Geometry: final body of the model. Coordinates: model frame, mm. Give positions to 0.01 mm unless a question says otherwise; leave off trailing zeros. Write each loop counter-clockwise with the first axis right and the second up, starting at its lowest first coordinate (ties: lowest second). Pieces come first, ordered by that corner, then holes. Notation, with made-up numbers: M 62.25,70 L 104.25,70 A30 ccw 104.25,104 Z; hole C 18,-12 d5. An arc over 180 degrees is marked long. One line per question, with ' | ' between items.
from build123d import *

# Parameters (mm, degrees)
F0_W     = 100
F0_H     = 120
F0_R     = 2
F1_DEPTH = 2
F3_DEPTH = 25
F4_R     = 1.5
F5_DEPTH = 2.001


with BuildPart() as f1:
    # F0 (on Front) → F1 (new body)
    with BuildSketch(Plane.XZ):
        Rectangle(F0_W, F0_H)
        with Locations((-40, -50)):
            Circle(F0_R, mode=Mode.SUBTRACT)
        with Locations((40, -50)):
            Circle(F0_R, mode=Mode.SUBTRACT)
        with Locations((-40, 50)):
            Circle(F0_R, mode=Mode.SUBTRACT)
        with Locations((40, 50)):
            Circle(F0_R, mode=Mode.SUBTRACT)
    extrude(amount=F1_DEPTH)

    # F2 (on face) → F3 (cut)
    with BuildSketch(Plane.XZ.offset(2)):
        with BuildLine():
            Line((-1.25, 21.980018), (-9.75, 17.072541))
            ThreePointArc((-9.75, 17.072541), (-10.665064, 16.157477), (-11, 14.907477))
            Line((-11, 14.907477), (-11, 5.092523))
            ThreePointArc((-11, 5.092523), (-10.665064, 3.842523), (-9.75, 2.927459))
            Line((-9.75, 2.927459), (-1.25, -1.980018))
            ThreePointArc((-1.25, -1.980018), (0, -2.314955), (1.25, -1.980018))
            Line((1.25, -1.980018), (9.75, 2.927459))
            ThreePointArc((9.75, 2.927459), (10.665064, 3.842523), (11, 5.092523))
            Line((11, 5.092523), (11, 10.354255))
            Line((11, 10.354255), (0, 10.354255))
            Line((0, 10.354255), (0, 22.314955))
            ThreePointArc((0, 22.314955), (-0.647048, 22.229769), (-1.25, 21.980018))
        make_face()
        with BuildLine():
            ThreePointArc((1.25, 21.980018), (0.647048, 22.229769), (0, 22.314955))
            Line((0, 22.314955), (0, 10.354255))
            Line((0, 10.354255), (11, 10.354255))
            Line((11, 10.354255), (11, 14.907477))
            ThreePointArc((11, 14.907477), (10.665064, 16.157477), (9.75, 17.072541))
            Line((9.75, 17.072541), (1.25, 21.980018))
        make_face()
    extrude(amount=-F3_DEPTH, mode=Mode.SUBTRACT)

    # F4 (on face) → F5 (cut, through all)
    with BuildSketch(Plane.XZ.offset(2)):
        with Locations((3.75, 47.5)):
            Circle(F4_R)
        with Locations((3.75, 40)):
            Circle(F4_R)
        with Locations((3.75, 32.5)):
            Circle(F4_R)
        with Locations((11.25, 47.5)):
            Circle(F4_R)
        with Locations((11.25, 40)):
            Circle(F4_R)
        with Locations((11.25, 32.5)):
            Circle(F4_R)
        with Locations((11.25, 25)):
            Circle(F4_R)
        with Locations((18.75, 47.5)):
            Circle(F4_R)
        with Locations((18.75, 40)):
            Circle(F4_R)
        with Locations((18.75, 32.5)):
            Circle(F4_R)
        with Locations((18.75, 25)):
            Circle(F4_R)
        with Locations((18.75, 17.5)):
            Circle(F4_R)
        with Locations((18.75, 10)):
            Circle(F4_R)
        with Locations((18.75, 2.5)):
            Circle(F4_R)
        with Locations((26.25, 47.5)):
            Circle(F4_R)
        with Locations((26.25, 40)):
            Circle(F4_R)
        with Locations((26.25, 32.5)):
            Circle(F4_R)
        with Locations((26.25, 25)):
            Circle(F4_R)
        with Locations((26.25, 17.5)):
            Circle(F4_R)
        with Locations((26.25, 10)):
            Circle(F4_R)
        with Locations((26.25, 2.5)):
            Circle(F4_R)
        with Locations((3.75, -12.5)):
            Circle(F4_R)
        with Locations((3.75, -20)):
            Circle(F4_R)
        with Locations((3.75, -27.5)):
            Circle(F4_R)
        with Locations((3.75, -35)):
            Circle(F4_R)
        with Locations((11.25, -5)):
            Circle(F4_R)
        with Locations((11.25, -12.5)):
            Circle(F4_R)
        with Locations((11.25, -20)):
            Circle(F4_R)
        with Locations((11.25, -27.5)):
            Circle(F4_R)
        with Locations((11.25, -35)):
            Circle(F4_R)
        with Locations((18.75, -5)):
            Circle(F4_R)
        with Locations((18.75, -12.5)):
            Circle(F4_R)
        with Locations((18.75, -20)):
            Circle(F4_R)
        with Locations((18.75, -27.5)):
            Circle(F4_R)
        with Locations((26.25, -5)):
            Circle(F4_R)
        with Locations((26.25, -12.5)):
            Circle(F4_R)
        with Locations((26.25, -20)):
            Circle(F4_R)
        with Locations((-3.75, 47.5)):
            Circle(F4_R)
        with Locations((-3.75, 40)):
            Circle(F4_R)
        with Locations((-3.75, -12.5)):
            Circle(F4_R)
        with Locations((-3.75, -35)):
            Circle(F4_R)
        with Locations((-26.25, 17.5)):
            Circle(F4_R)
        with Locations((-26.25, -12.5)):
            Circle(F4_R)
        with Locations((-26.25, -5)):
            Circle(F4_R)
        with Locations((-26.25, 47.5)):
            Circle(F4_R)
        with Locations((-26.25, 32.5)):
            Circle(F4_R)
        with Locations((-26.25, 10)):
            Circle(F4_R)
        with Locations((-26.25, 40)):
            Circle(F4_R)
        with Locations((-3.75, -27.5)):
            Circle(F4_R)
        with Locations((-11.25, 40)):
            Circle(F4_R)
        with Locations((-26.25, 2.5)):
            Circle(F4_R)
        with Locations((-11.25, -27.5)):
            Circle(F4_R)
        with Locations((-11.25, 32.5)):
            Circle(F4_R)
        with Locations((-11.25, 47.5)):
            Circle(F4_R)
        with Locations((-18.75, 25)):
            Circle(F4_R)
        with Locations((-18.75, 10)):
            Circle(F4_R)
        with Locations((-11.25, -35)):
            Circle(F4_R)
        with Locations((-11.25, -20)):
            Circle(F4_R)
        with Locations((-18.75, 2.5)):
            Circle(F4_R)
        with Locations((-18.75, -12.5)):
            Circle(F4_R)
        with Locations((-11.25, -5)):
            Circle(F4_R)
        with Locations((-11.25, -12.5)):
            Circle(F4_R)
        with Locations((-18.75, -20)):
            Circle(F4_R)
        with Locations((-18.75, 32.5)):
            Circle(F4_R)
        with Locations((-26.25, 25)):
            Circle(F4_R)
        with Locations((-26.25, -20)):
            Circle(F4_R)
        with Locations((-11.25, 25)):
            Circle(F4_R)
        with Locations((-3.75, 32.5)):
            Circle(F4_R)
        with Locations((-18.75, 47.5)):
            Circle(F4_R)
        with Locations((-18.75, -5)):
            Circle(F4_R)
        with Locations((-18.75, 40)):
            Circle(F4_R)
        with Locations((-18.75, -27.5)):
            Circle(F4_R)
        with Locations((-18.75, 17.5)):
            Circle(F4_R)
        with Locations((-3.75, -20)):
            Circle(F4_R)
    extrude(amount=-F5_DEPTH, mode=Mode.SUBTRACT)


solid = f1.part
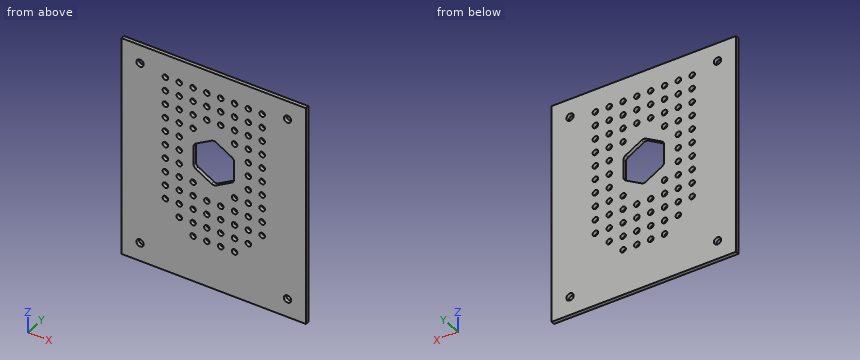
(1) First-contact query: P1, Ø2.5, axis at x = -3.75, z = -20, coming from the +Y side. Flat tip, straight axial feed; report the tip coordinate or a pass-through.
Working result:
P1: passes through
(2) Cut plane C-C, the plane x = 40. Return loops of the section in (y, z), then the cut area to 3 significant figures.
Working result:
outline: M -2,-60 L 0,-60 L 0,-52 L -2,-52 Z; M -2,-48 L 0,-48 L 0,48 L -2,48 Z; M -2,52 L 0,52 L 0,60 L -2,60 Z | area: 224 mm^2
(3) Cut plane B-B, the plane z = -50. Return loops of the section in (x, y).
Working result:
outline: M -50,-2 L -42,-2 L -42,0 L -50,0 Z; M -38,-2 L 38,-2 L 38,0 L -38,0 Z; M 42,-2 L 50,-2 L 50,0 L 42,0 Z
(4) Cut plane D-D, the plane z = -35. Return loops of the section in (x, y).
Working result:
outline: M -50,-2 L -12.75,-2 L -12.75,0 L -50,0 Z; M -9.75,-2 L -5.25,-2 L -5.25,0 L -9.75,0 Z; M -2.25,-2 L 2.25,-2 L 2.25,0 L -2.25,0 Z; M 5.25,-2 L 9.75,-2 L 9.75,0 L 5.25,0 Z; M 12.75,-2 L 50,-2 L 50,0 L 12.75,0 Z
(5) Material intervals for L1, parallel to X at y = -1.4, z = -49; L2, parallel to Z at x = 1.5, y = -1.6; L3, parallel to X at y = -0.4, z = 2, sorted ascending. Write a range as [from, to].
Working result:
L1: x = [-50, -41.73], [-38.27, 38.27], [41.73, 50] | L2: z = [-60, -1.84], [21.84, 60] | L3: x = [-50, -27.66], [-24.84, -20.16], [-17.34, -8.14], [8.14, 17.34], [20.16, 24.84], [27.66, 50]
(6) Cut plane A-A, the plane z = 25. Return loops of the section in (x, y).
Working result:
outline: M -50,-2 L -27.75,-2 L -27.75,0 L -50,0 Z; M -24.75,-2 L -20.25,-2 L -20.25,0 L -24.75,0 Z; M -17.25,-2 L -12.75,-2 L -12.75,0 L -17.25,0 Z; M -9.75,-2 L 9.75,-2 L 9.75,0 L -9.75,0 Z; M 12.75,-2 L 17.25,-2 L 17.25,0 L 12.75,0 Z; M 20.25,-2 L 24.75,-2 L 24.75,0 L 20.25,0 Z; M 27.75,-2 L 50,-2 L 50,0 L 27.75,0 Z
